For this review, take the finished solid that the model builds, in its own axes (mm). Give positions to 0.01 mm unless a question says otherwise; leave off trailing zeros. Loops run counter-clockwise (first coordinate to the right, second up) from the corner with the lowest first, then second, coordinate; pieces in that order, holes last. Notation, with made-up numbers: (32, -15.5) -> (81, -15.5) arc R21 ccw to (81, -6.5) -> close; hole circle Ø6 at (35, -14). An arc over 180 degrees is marked (long way). One line per question, with ' | ' between items. Start each with the question number.
(1) Consider section C-C (z = 0.3). Write out the cut boundary in (x, y), and give its area (3 significant figures).
(2) Draft analysis for pull direction X (two halves, no side actions). For faces 1 (the cylindrical face through (-4.075, 31.034, 0.887)), 2 (the flat face through (-0.1, 25.5, 2)), 3 (the cylindrical face through (23.846, 7.509, 0.913)), state which applies: +X half, -X half, draft (parallel to the pull), parting line (faces both ways), or undercut.
(3) Consider section A-A (y = 0). Write out the cut boundary in (x, z).
(4) Insertion check: P1, Ø1, axis at x = -1, z = 1, coming from the +Y side; P2, Ø12, axis at x = 15.5, y = 9, coming from the -Z side. Each pin has a flat end and moves straight along its axis. Give the tip position at first contact, or say it passes through.
(5) Wall thickness on probe 1 along Y at (x, z) = (0, 0.8); probe 2 along Y at (x, z) = (-17.5, 1.6); probe 3 along X at (y, z) = (18, 1.25): over which ranges is each line inside the solid? List them lowest first.
from build123d import *

# Parameters (mm, degrees)
F0_R     = 31.3
F1_DEPTH = 2
F2_R     = 25
F3_DEPTH = 2
F4_R     = 0.2


with BuildPart() as f1:
    # F0 (on Top) → F1 (new body)
    with BuildSketch(Plane.XY):
        Circle(F0_R)
    extrude(amount=F1_DEPTH)

    # F2 (on face) → F3 (cut)
    with BuildSketch(Plane.XY.offset(2)):
        Circle(F2_R)
    extrude(amount=-F3_DEPTH, mode=Mode.SUBTRACT)

    # F4
    f4_edges = [f1.edges().sort_by_distance(p)[0] for p in [
        (-31.3, 0, 2),
        (-25, 0, 2),
    ]]
    fillet(f4_edges, radius=F4_R)


solid = f1.part
A:
1) outline: circle Ø62.6 at (0, 0); hole circle Ø50 at (0, 0) | area: 1,110 mm^2
2) face 1: parting line | face 2: draft | face 3: undercut
3) outline: (-31.3, 0) -> (-25, 0) -> (-25, 1.8) arc R0.2 ccw to (-25.2, 2) -> (-31.1, 2) arc R0.2 ccw to (-31.3, 1.8) -> close; (25, 0) -> (31.3, 0) -> (31.3, 1.8) arc R0.2 ccw to (31.1, 2) -> (25.2, 2) arc R0.2 ccw to (25, 1.8) -> close
4) P1: stops at y = 31.3 | P2: passes through
5) probe 1: y = -31.3 to -25, 25 to 31.3 | probe 2: y = -25.95 to -17.85, 17.85 to 25.95 | probe 3: x = -25.61 to -17.35, 17.35 to 25.61
